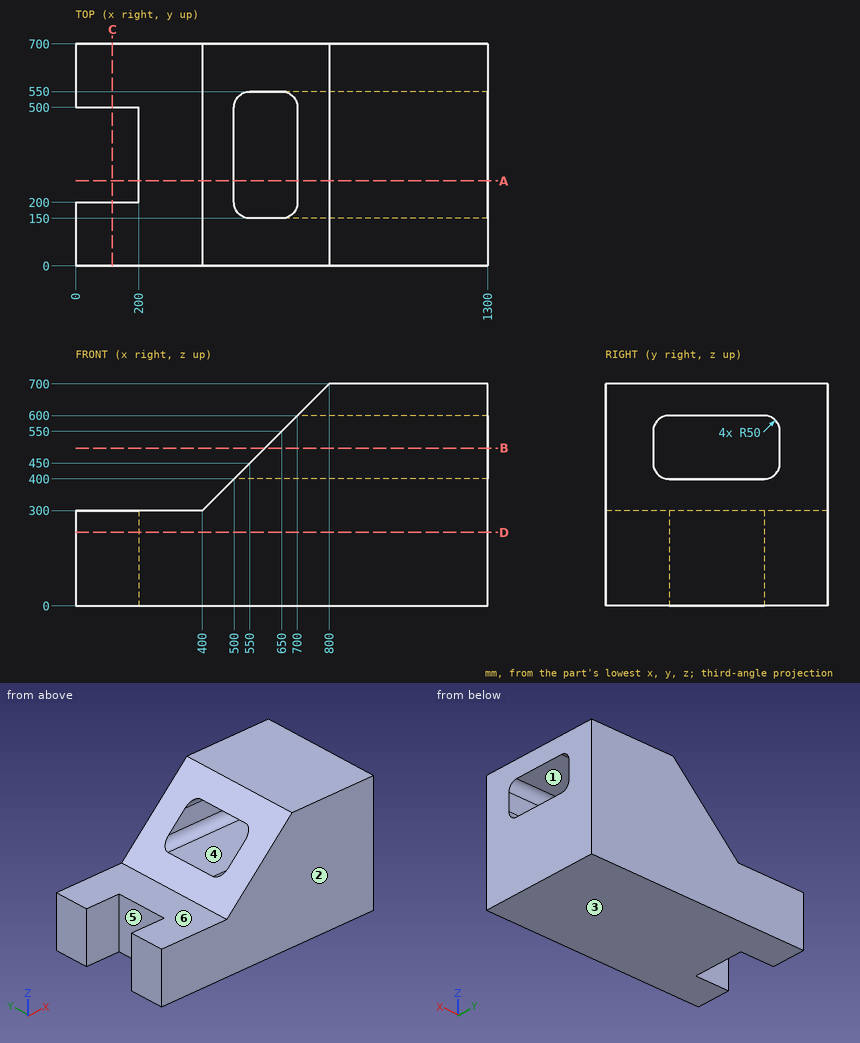
Drawing for the job (mm, zero at the part's lowest x, y, z). A direction names the side the tool comes from. Give positions to 0.01 mm unless a question says otherwise; leave off trailing zeros. Order: outer loops, then holes, each group sorted by start corner. A loop starts at its lowest first (then second) coordinate and runs counter-clockwise, first axis right, second up. Notation, with made-up numbers: M -11,4.25 L 14,4.25 A24 ccw 14,15.25 Z; hole C -16,-9.5 d8. An arc over 180 degrees is marked long. Use a Markdown table: item, result. Add a question column.
(1) 3-axis set-ups, long thin cutter, end or side, ignore diameter. For the marked faces 4, 5 and 6: which of +Z, -Z, +X, -X, +Y, -Y reach the whole face in a straight line?
(2) Saw through at B-B, the plane z = 497.5. Give the cut face in (x, y).
(3) Saw through at A-A, the plane y = 268. Give the cut face in (x, z), and give its area (3 significant figures).
(4) Saw through at D-D, the plane z = 231.5. Give the cut face in (x, y).
(5) Saw through at C-C, the plane x = 116.5. Give the cut face in (y, z), and give its area (3 significant figures).
(6) Drop flat-ended pins along their axis: P1, Ø3, axis at x = 327.5, y = 338.5, coming from the +Z side; P2, Ø2, axis at x = 608, y = 324.5, coming from the +Z side. Give the stop position or say it passes through.
(7) Mould opens along Y. For the marked faces 1, 2 and 3 say: +Y half, -Y half, draft (parallel to the pull), parting line (faces both ways), or undercut.
(8) Probe line 1 along Y through (x, z) = (1158.5, 512); line 2 along Z through (x, y) = (1019, 215.5); line 3 along X through (y, z) = (272, 74). List the from-to ranges inside material, lowest first. Write a range as [from, to].
Answer key:
| question | item | result |
|---|---|---|
| 1 | face 4 | +X, -X |
| 1 | face 5 | +Z, -Z, -X |
| 1 | face 6 | +Z, -X, +Y, -Y |
| 2 | outline | M 597.5,0 L 1300,0 L 1300,150 L 597.5,150 Z; M 597.5,550 L 1300,550 L 1300,700 L 597.5,700 Z |
| 3 | outline | M 200,0 L 1300,0 L 1300,400 L 500,400 L 400,300 L 200,300 Z; M 700,600 L 1300,600 L 1300,700 L 800,700 Z |
| 3 | area | 470,000 mm^2 |
| 4 | outline | M 0,0 L 1300,0 L 1300,700 L 0,700 L 0,500 L 200,500 L 200,200 L 0,200 Z |
| 5 | outline | M 0,0 L 200,0 L 200,300 L 0,300 Z; M 500,0 L 700,0 L 700,300 L 500,300 Z |
| 5 | area | 120,000 mm^2 |
| 6 | P1 | z = 300 |
| 6 | P2 | z = 400 |
| 7 | face 1 | undercut |
| 7 | face 2 | -Y half |
| 7 | face 3 | draft |
| 8 | line 1 | [0, 150], [550, 700] |
| 8 | line 2 | [0, 400], [600, 700] |
| 8 | line 3 | [200, 1300] |
